```python
from build123d import *

# Parameters (mm, degrees)
F0_W      = 101.6
F0_H      = 76.2
F1_DEPTH  = 6.35
F3_DEPTH  = 5.334
F4_DEPTH  = 12.7
F5_R      = 5.08
F6_SIZE   = 5.08
F8_T      = -2.54
F9_D      = 12.7
F10_R     = 9.3699791153
F11_DEPTH = 10.16
F12_R     = 5.08
F13_W     = 10.32633055
F13_H     = 4.7064404935
F14_DEPTH = 25.4


with BuildPart() as f1:
    # F0 (on Top) → F1 (new body)
    with BuildSketch(Plane.XY):
        with Locations((-0.1408625394, -1.77114314)):
            Rectangle(F0_W, F0_H)
    extrude(amount=F1_DEPTH)

    # F3 (add): a face of the model
    f3_faces = [f1.faces().sort_by_distance(p)[0] for p in [
        (-0.1408625394, -1.77114314, 0),
    ]]
    extrude(f3_faces, amount=-F3_DEPTH)

    # F2 (on face) → F4 (join)
    with BuildSketch(Plane.XY.offset(6.35)):
        with BuildLine():
            Line((-37.6103334129, -16.3400694728), (-37.6103334129, -39.87114314))
            Line((-37.6103334129, -39.87114314), (50.6591374606, -39.87114314))
            Line((50.6591374606, -39.87114314), (50.6591374606, 29.5811630785))
            Line((50.6591374606, 29.5811630785), (25.4961457103, 29.5811630785))
            ThreePointArc((25.4961457103, 29.5811630785), (7.7217190937, -12.3147544324), (-37.6103334129, -16.3400694728))
        make_face()
    extrude(amount=F4_DEPTH)

    # F5
    f5_edges = [f1.edges().sort_by_distance(p)[0] for p in [
        (-0.140863, 36.328857, 6.35),
    ]]
    fillet(f5_edges, radius=F5_R)

    # F6
    f6_edges = [f1.edges().sort_by_distance(p)[0] for p in [
        (50.659137, -5.14499, 19.05),
    ]]
    chamfer(f6_edges, length=F6_SIZE)

    # F8
    f8_openings = [f1.faces().sort_by_distance(p)[0] for p in [
        (-0.140863, -1.771143, 0),
    ]]
    offset(amount=F8_T, openings=f8_openings, kind=Kind.INTERSECTION)

    # F9 (through all)
    with Locations(Plane.XY.offset(6.35)):
        with Locations((-26.9047711045, 0)):
            Hole(F9_D / 2)

    # F10 (on face) → F11 (join)
    with BuildSketch(Plane.XY.offset(19.05)):
        with Locations((25.0284876674, -17.6028143615)):
            Circle(F10_R)
    extrude(amount=F11_DEPTH)

    # F12
    f12_edges = [f1.edges().sort_by_distance(p)[0] for p in [
        (15.658509, -17.602814, 29.21),
    ]]
    fillet(f12_edges, radius=F12_R)

    # F13 (on face) → F14 (cut)
    with BuildSketch(Plane.XY.offset(19.05)):
        with Locations((-5.163165275, -30.2898483351)):
            Rectangle(F13_W, F13_H)
    extrude(amount=-F14_DEPTH, mode=Mode.SUBTRACT)


solid = f1.part
```
For this review, take the finished solid that the model builds, in its own axes (mm). A direction names the side the tool comes from. Coordinates: 2 decimals unless noted, no trailing zeros. Order: outer loops, then holes, each group sorted by start corner. A loop starts at its lowest first (then second) coordinate and runs counter-clockwise, first axis right, second up. Notation, with made-up numbers: (75.5, -32.75) -> (98.5, -32.75) arc R30 cw to (98.5, -8.75) -> close; hole circle Ø5 at (12.25, -10). An arc over 180 degrees is marked (long way). Use CSV: the item, a comma, the result in double quotes. Start each with the question number.
Item 1: Wall thickness on probe 1 along Y at (x, z) = (35, 5.25); probe 2 along Y at (x, z) = (3, 1.5); probe 3 along X at (y, z) = (5, 4): over which ranges is each line inside the solid? List them lowest first.
Item 2: We need section A-A, the plane z = 10. Give the boundary of the cut face in (x, y), then the cut area to 3 significant figures.
Item 3: Draft analysis for pull direction X (two halves, no side actions). For faces 1 (the face through (-35.07, -29, 10)), 2 (the face through (-50.941, -2, 3)), 3 (the face through (25, -18, 29.21)), state which applies: pulls with the +X half, pulls with the -X half, needs draft (parallel to the pull), parting line crosses it, or undercut.
Item 4: We need section B-B, the plane y = 0. Give the boundary of the cut face in (x, z), then the cut area to 3 significant figures.
Item 5: Insertion check: pin 1 (4 mm diameter, centred on x = 33, z = 11.5, fed in from +Y); pin 2 (20.5 mm diameter, centred on x = 2.5, y = -19.5, fed in from -Z); pin 3 (2 mm diameter, centred on x = -38.5, y = -30.5, fed in from +Z); pin 4 (11.5 mm diameter, centred on x = -26.9, y = 0, fed in from +Z) (1 decimal). Each pin has a flat end and moves straight along its axis. Give the tip position at first contact, or say it passes through.
Item 6: We need section C-C, the plane x = -44. Give the boundary of the cut face in (y, z).
Item 7: We need section D-D, the plane x = 14. Give the boundary of the cut face in (y, z).
Item 8: For faces 4 (the face through (48.119, -2, 6)), 5 (the face through (38, 29.581, 13)), 6 (the face through (-5, -32.643, 18)), list the 3-axis set-ups (+Z, -Z, +X, -X, +Y, -Y) from which the entire face can be reached by the end or side of a thin tool; tool diameter is ignored.
Derived:
1,probe 1,"y = -39.87 to -37.33, 27.04 to 34.41"
1,probe 2,"y = -39.87 to -37.33, 33.78 to 36.32"
1,probe 3,"x = -50.94 to -30.82, -22.99 to 24.67, 48.12 to 50.66"
2,outline,"(-37.61, -39.87) -> (50.66, -39.87) -> (50.66, 29.58) -> (25.5, 29.58) arc R44.22 cw to (-37.61, -16.34) -> close; hole (-35.07, -37.33) -> (48.12, -37.33) -> (48.12, 27.04) -> (28.33, 27.04) arc R46.76 cw to (-35.07, -20.21) -> close"
2,area,"737 mm^2"
3,face 1,"undercut"
3,face 2,"pulls with the -X half"
3,face 3,"needs draft"
4,outline,"(-50.94, 0) -> (-48.4, 0) -> (-48.4, 3.81) -> (-33.25, 3.81) -> (-33.25, 6.35) -> (-50.94, 6.35) -> close; (-20.55, 3.81) -> (22.16, 3.81) -> (22.16, 16.51) -> (44.53, 16.51) -> (48.12, 12.92) -> (48.12, 0) -> (50.66, 0) -> (50.66, 13.97) -> (45.58, 19.05) -> (19.2, 19.05) -> (19.2, 6.35) -> (-20.55, 6.35) -> close"
4,area,"309 mm^2"
5,pin 1,"stops at y = 29.58"
5,pin 2,"stops at z = 3.81"
5,pin 3,"stops at z = 19.05"
5,pin 4,"passes through"
6,outline,"(-39.87, 0) -> (-37.33, 0) -> (-37.33, 3.81) -> (31.25, 3.81) arc R2.54 cw to (33.79, 1.27) -> (33.79, 0) -> (36.33, 0) -> (36.33, 1.27) arc R5.08 ccw to (31.25, 6.35) -> (-39.87, 6.35) -> close"
7,outline,"(-39.87, 0) -> (-37.33, 0) -> (-37.33, 16.51) -> (-10.37, 16.51) -> (-10.37, 3.81) -> (31.25, 3.81) arc R2.54 cw to (33.79, 1.27) -> (33.79, 0) -> (36.33, 0) -> (36.33, 1.27) arc R5.08 ccw to (31.25, 6.35) -> (-6.76, 6.35) -> (-6.76, 19.05) -> (-39.87, 19.05) -> close"
8,face 4,"-Z"
8,face 5,"+Z, +X, -X, +Y"
8,face 6,"+Z, -Z"
